Verification items for this drawing (mm, ordinates from the low corner). Give positions to 0.01 mm unless a question says otherwise; leave off trailing zeros. Write each question's results on one line, items separated by ' | '. Start each with the question number.
1) Scan line: line 1 (Y direction, x = 29, z = 23). Record every from-to range of solid material in increasing order. Write a range as from..to.
2) Draft check along X on the marked faces 1, 2 and 3. Enter one of: pulls with the +X half, pulls with the -X half, needs draft (parallel to the pull), parting line crosses it, or undercut.
3) Depth check by flat-ended pin: pin 1 (8 mm diameter, centred on x = 31.5, y = 140, fed in from -Z). Enter the tip coordinate at first touch or a pass-through.
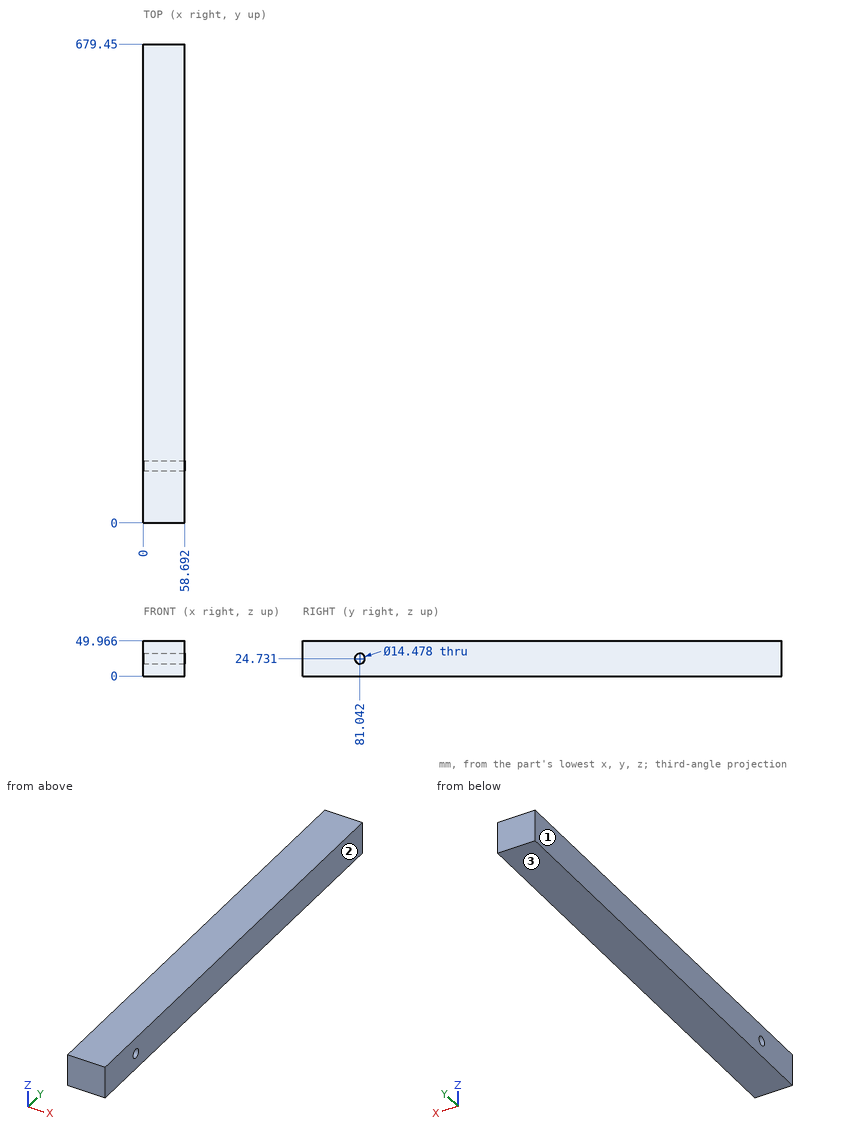
Result:
1) line 1: 0..74.01, 88.07..679.45
2) face 1: pulls with the -X half | face 2: pulls with the +X half | face 3: needs draft
3) pin 1: z = 0
